Work out the finished part from the listing and answer in its coordinate system (mm). A direction names the side the tool comes from. Coordinates: 2 decimals unless noted, no trailing zeros. Write each loop counter-clockwise with the first axis right and the second up, starting at its lowest first coordinate (ties: lowest second). Pieces come first, ordered by that corner, then holes. Notation, with made-up numbers: (21, 49.5) - (30, 49.5) arc R15 cw to (30, 78.5) - close; hole circle Ø5 at (56, -23.5). An arc over 180 degrees is marked (long way). Use a Markdown table: item, result. Add a question column.
(1) The part is cut by section A-A, the plane z = 16.5. Give the vertices of the cut face in (x, y), then the cut area to 3 significant figures.
(2) Given pin 1 Ø0.8 at (y, z) = (-0.5, 21) entering from +X; pin 2 Ø2 at (x, z) = (8.5, 20.5) entering from -Y; pin 3 Ø3 at (y, z) = (-3, 26.5) entering from -X, each flat-ended and moving along its own axis, determine where each tip first touches the part or whether it passes through.
(3) The part is cut by section B-B, the plane x = 8.5. Give the vertices of the cut face in (y, z).
(4) A tool of negligible diameter and unlimited length cuts with its end or side. For faces 1 (the face through (-12.003, -3, 22)), 2 (the face through (-11, -2.21, 22)), 3 (the face through (5.597, -3, 22)), 4 (the face through (3.047, -1, 22)), from which of +Z, -Z, +X, -X, +Y, -Y can it reach the whole face along a straight path? Write none if from no direction.
(5) For a pull along X with two mould halves and no side action, classify faces 5 (the face through (4, -2.21, 22)), 6 (the face through (-3.05, -3.62, 32.12)), 7 (the face through (-19.203, 2, 19)) as released by +X, released by -X, zero draft, split by the parting line, or undercut.
(6) Find the intervals of material crossed by line 1 (Y direction, x = -17, z = 4); line 2 (Z direction, x = -13, y = -3); line 3 (X direction, y = -1.5, z = 42.5), in increasing order. Write a range as from..to.
from build123d import *

# Parameters (mm, degrees)
SKETCH1_W           = 6.25
SKETCH1_H           = 2.5
SKETCH1_W_2         = 8.8
BOSS_EXTRUDE1_DEPTH = 45
SKETCH9_W           = 32
SKETCH9_H           = 7.5
BOSS_EXTRUDE3_DEPTH = 3


with BuildPart() as part:
    # Sketch1 → Boss-Extrude1 (new body)
    with BuildSketch(Plane.XY):
        Polygon((-3.202898551, 2.789855072), (-3.202898551, 0.289855072), (3.047101449, 0.289855072), (12.797101449, 0.289855072), (12.797101449, 2.789855072), align=None)
        with Locations((-0.077898551, -0.960144928)):
            Rectangle(SKETCH1_W, SKETCH1_H)
        with Locations((1.197101449, -3.460144928)):
            Rectangle(SKETCH1_W_2, SKETCH1_H)
    boss_extrude1 = extrude(amount=BOSS_EXTRUDE1_DEPTH)

    # Mirror1: Boss-Extrude1 across plane
    add(boss_extrude1.mirror(Plane(origin=(-3.202898551, 0, 45), x_dir=(0, 0, 1), z_dir=(-1, 0, 0))))

    # Cut-Extrude2 cone 1 section (through the dimple's axis) → Cut-Extrude2 (revolve, cut)
    with BuildSketch(Plane(origin=(-3.202898551, -4.710144928, 32.5), x_dir=(0, 0, -1), z_dir=(1, 0, 0))):
        Polygon((0, 0), (1.5, 0), (0, 1.5), align=None)
    revolve(axis=Axis((-3.202898551, -4.710144928, 32.5), (0, 1, 0)), mode=Mode.SUBTRACT)

    # Cut-Extrude2 cone 2 section (through the dimple's axis) → Cut-Extrude2 cone 2 (revolve, cut)
    with BuildSketch(Plane(origin=(-3.202898551, -4.710144928, 12.5), x_dir=(0, 0, -1), z_dir=(1, 0, 0))):
        Polygon((0, 0), (1.5, 0), (0, 1.5), align=None)
    revolve(axis=Axis((-3.202898551, -4.710144928, 12.5), (0, 1, 0)), mode=Mode.SUBTRACT)

    # Sketch9 → Boss-Extrude3 (add)
    with BuildSketch(Plane(origin=(0, 0, 0), x_dir=(-1, 0, 0), z_dir=(0, 0, -1))):
        with Locations((3.202898551, -0.960144928)):
            Rectangle(SKETCH9_W, SKETCH9_H)
    extrude(amount=BOSS_EXTRUDE3_DEPTH)


solid = part.part
Model answer:
| question | item | result |
|---|---|---|
| 1 | outline | (-19.2, 0.29) - (-9.45, 0.29) - (-9.45, -2.21) - (-12, -2.21) - (-12, -4.71) - (5.6, -4.71) - (5.6, -2.21) - (3.05, -2.21) - (3.05, 0.29) - (12.8, 0.29) - (12.8, 2.79) - (-19.2, 2.79) - close |
| 1 | area | 155 mm^2 |
| 2 | pin 1 | x = 3.05 |
| 2 | pin 2 | y = 0.29 |
| 2 | pin 3 | x = -12 |
| 3 | outline | (-4.71, -3) - (2.79, -3) - (2.79, 45) - (0.29, 45) - (0.29, 0) - (-4.71, 0) - close |
| 4 | face 1 | +Z, -X, -Y |
| 4 | face 2 | +Z, -X |
| 4 | face 3 | +Z, +X, -Y |
| 4 | face 4 | +Z, +X |
| 5 | face 5 | zero draft |
| 5 | face 6 | undercut |
| 5 | face 7 | released by -X |
| 6 | line 1 | 0.29..2.79 |
| 6 | line 2 | -3..0 |
| 6 | line 3 | -9.45..3.05 |
